```python
from build123d import *

# Parameters (mm, degrees)
F0_R     = 609.6
F1_DEPTH = 1873.25
F4_DEPTH = 304.8


# Not quite as in the source:
# - a feature of the source that left no trace in its solid (it failed there, or was rolled back) is left out
# - a pattern or mirror of a feature is missing from the dataset's text; its kind, count and spacing are read off the source's solid


with BuildPart() as f1:
    # F0 (on Front) → F1 (new body)
    with BuildSketch(Plane.XZ):
        Circle(F0_R)
    extrude(amount=-F1_DEPTH)

    # F1_copies: F1 across plane


with BuildPart() as f1_1:
    add(f1.part)
    add(f1.part.mirror(Plane(origin=(0, 930.275, 0), x_dir=(0, 0, -1), z_dir=(0, -1, 0))))

    # F3 (on offset) → F4 (join)
    with BuildSketch(Plane.XZ.offset(-149.225)):
        with BuildLine():
            Line((-384.175, -473.3093379334), (-384.175, -800.1))
            Line((-384.175, -800.1), (-168.275, -800.1))
            Line((-168.275, -800.1), (-168.275, -585.9144002113))
            ThreePointArc((-168.275, -585.9144002113), (-170.6576627394, -585.2248475145), (-173.0375, -584.5256055929))
            Line((-173.0375, -584.5256055929), (-173.0375, -795.3375))
            Line((-173.0375, -795.3375), (-379.4125, -795.3375))
            Line((-379.4125, -795.3375), (-379.4125, -477.1355308964))
            ThreePointArc((-379.4125, -477.1355308964), (-381.7985430528, -475.2284003748), (-384.175, -473.3093379334))
        make_face()
    f4 = extrude(amount=-F4_DEPTH)

    # F4_copies: F4 across plane
    add(f4.mirror(Plane.ZX.offset(930.275)))

    # F5: F1 across plane


with BuildPart() as f1_2:
    add(f1_1.part)
    add(f1_1.part.mirror(Plane.YZ))


solid = f1_2.part
```
Design review of the part built by this model. Coordinates are the model's own, in mm. A direction names the side the tool comes from. Coordinates: 2 decimals unless noted, no trailing zeros. Write each loop counter-clockwise with the first axis right and the second up, starting at its lowest first coordinate (ties: lowest second). Pieces come first, ordered by that corner, then holes.
1) Insertion check: pin 1 (1 mm diameter, centred on y = 1360.5, z = -456, fed in from -X); pin 2 (3 mm diameter, centred on y = 755.5, z = -511, fed in from +X); pin 3 (6 mm diameter, centred on x = -470.5, y = 1565, fed in from -Z). Each pin has a flat end and moves straight along its axis. Give the tip position at first contact, or say it passes through.
2) Machinability: for faces 4 (the flat face through (381, 454.025, -660)), 5 (the flat face through (381, 149.225, -660)), 6 (the flat face through (-275, 299, -795.338)), 7 (the flat face through (-381, 1711.325, -660)), which of the approach directions +Z, -Z, +X, -X, +Y, -Y give a long, thin tool a straight path to every point of the face, cutting with its end or side? Answer none if there is none.
3) Mouldability with a two-part tool opening along X and no side actions: class faces 1 (the flat face through (-384.175, 299, -634)), 2 (the flat face through (-381, 149.225, -660)), 3 (the flat face through (275, 1561, -795.338)) as +X half, -X half, draft (parallel to the pull), parting line (faces both ways), or undercut.
4) Add section B-B (z = -510.5). State how many separate pieces and enclosed holes the cut face has, plus the area to 3 significant figures.
5) To check wall thickness, follow L1, parallel to X at y = 1413, z = -536 (1 decimal); L2, parallel to Z at x = -11, y = 1719; L3, parallel to Z at x = 192, y = 1692.5. State the ranges of each line that lie inside material, in increasing order.
6) Add section A-A (y = 1688). Write out the cut boundary in (x, z) (1 decimal), plus the area to 3 significant figures.
7) Add section D-D (y = 1348). Write out the cut boundary in (x, z).
8) Add section C-C (x = 0). Write out the cut boundary in (y, z), plus the area to 3 significant figures.
Check result:
1. pin 1: stops at x = -405.13
1. pin 2: stops at x = 334.7
1. pin 3: stops at z = -391.22
2. face 4: -Z, +X
2. face 5: -Z, +X, -Y
2. face 6: +Y, -Y
2. face 7: -Z, -X, +Y
3. face 1: -X half
3. face 2: draft
3. face 3: undercut
4. separate pieces: 5
4. enclosed holes: 0
4. area: 1,260,000 mm2
5. L1: x = -384.2 to -379.4, -290.4 to 290.4, 379.4 to 384.2
5. L2: z = -609.5 to 609.5
5. L3: z = -800.1 to -795.34, -578.57 to 578.57
6. outline: (-384.2, -800.1) - (-168.3, -800.1) - (-168.3, -585.9) arc R609.6 ccw to (168.3, -585.9) - (168.3, -800.1) - (384.2, -800.1) - (384.2, -473.3) arc R609.6 ccw (long way) to (-384.2, -473.3) - close; hole (-379.4, -795.3) - (-173, -795.3) - (-173, -584.5) arc R609.6 cw to (-379.4, -477.1) - close; hole (173, -795.3) - (379.4, -795.3) - (379.4, -477.1) arc R609.6 cw to (173, -584.5) - close
6. area: 1,170,000 mm2
7. outline: circle Ø1219.2 at (0, 0)
8. outline: (-12.7, -609.6) - (1873.25, -609.6) - (1873.25, 609.6) - (-12.7, 609.6) - close
8. area: 2,300,000 mm2
